Source: CAD feature listing. Evaluate the final solid. Frame: model axes, mm. Give positions to 0.01 mm unless a question says otherwise; leave off trailing zeros. Order: outer loops, then holes, each group sorted by start corner. A loop starts at its lowest first (then second) coordinate and runs counter-clockwise, first axis right, second up. Notation, with made-up numbers: M -37.75,31.25 L -9.75,31.25 A18 cw -9.75,48.25 Z; hole C 60.5,48.5 d3. An arc over 180 degrees is marked long. Return JSON: item names as keys, results as strings.
Autodesk Inventor part; units mm, degrees
ref_plane "YZ Plane" through (0, 0, 0) normal (1, 0, 0) x (0, 1, 0)
ref_plane "XZ Plane" through (0, 0, 0) normal (0, 1, 0) x (-1, 0, 0)
ref_plane "XY Plane" through (0, 0, 0) normal (0, 0, 1) x (1, 0, 0)
sketch "Sketch1" plane through (0, 0, 0) normal (0, 1, 0) x (-1, 0, 0)
  line L0 (-3.175, -3.175) -> (3.175, -3.175)
  line L1 (3.175, -3.175) -> (3.175, 3.175)
  line L2 (3.175, 3.175) -> (-3.175, 3.175)
  line L3 (-3.175, 3.175) -> (-3.175, -3.175)
  line L4 (-3.175, -3.175) -> (3.175, 3.175) construction
  line L5 (3.175, -3.175) -> (-3.175, 3.175) construction
  point P0 (0, 0)
  dimension "d0" = 6.35
  dimension "d1" = 6.35
extrude "Extrusion1" add sketch "Sketch1" along normal blind 68.58
fillet "Fillet1" radius 1.5875 4 edges at (3.175, 34.29, 3.175) (3.175, 34.29, -3.175) (-3.175, 34.29, -3.175) (-3.175, 34.29, 3.175)
fillet "Fillet2" radius 0.7937 16 edges at (2.71, 0, -2.71) (0, 0, -3.175) (-2.71, 0, -2.71) (-3.175, 0, 0) (-2.71, 0, 2.71) (0, 0, 3.175) (2.71, 0, 2.71) (3.175, 0, 0) (2.71, 68.58, -2.71) (0, 68.58, -3.175) (-2.71, 68.58, -2.71) (-3.175, 68.58, 0) (-2.71, 68.58, 2.71) (0, 68.58, 3.175) (2.71, 68.58, 2.71) (3.175, 68.58, 0)
sketch "Sketch2" plane through (-1.5875, 67.7863, 3.175) normal (0, 0, 1) x (1, 0, 0)
  circle A0 centre (1.5875, -64.6113) radius 1.9844
  line L0 (0, -67.7863) -> (3.175, -67.7863)
  point P0 (1.5875, -67.7863)
  dimension "d6" = 3.9688
  dimension "d7" = 3.175
extrude "Extrusion2" cut sketch "Sketch2" against normal blind 50.8
sketch "Sketch3" plane through (-1.5875, 67.7863, 3.175) normal (0, 0, 1) x (1, 0, 0)
  circle A0 centre (1.5875, -23.7173) radius 1.9844
  arc A1 (3.175, -63.4206) -> (0, -63.4206) centre (1.5875, -64.6113) ccw
  point P0 (1.5875, -67.7863)
  dimension "d10" = 3.9688
  dimension "d11" = 40.894
extrude "Extrusion3" cut sketch "Sketch3" against normal blind 50.8
properties part number "wedgec" material "Stainless Steel"
1. Section query C-C (z = -0.5). Return loops of the section in (x, y) (3 decimals).
Evaluation:
{"outline": "M -3.175,0.794 A0.794 ccw -2.381,0 L 2.381,0 A0.794 ccw 3.175,0.794 L 3.175,67.786 A0.794 ccw 2.381,68.58 L -2.381,68.58 A0.794 ccw -3.175,67.786 Z; hole C 0,3.175 d3.969; hole C 0,44.069 d3.969"}
2. First-contact query: pin 1 (3 mm diameter, centred on x = -0.5, z = 0.5, fed in from -Y). Flat tip, straight axial feed; report the tip coordinate or a pass-through.
Evaluation:
{"pin 1": "stops at y = 0"}
3. Section query A-A (x = 0.5). Return loops of the section in (y, z) (3 decimals).
Evaluation:
{"outline": "M 0,-2.381 A0.794 ccw 0.794,-3.175 L 1.255,-3.175 L 1.255,3.175 L 0.794,3.175 A0.794 ccw 0,2.381 Z; M 5.095,-3.175 L 42.149,-3.175 L 42.149,3.175 L 5.095,3.175 Z; M 45.989,-3.175 L 67.786,-3.175 A0.794 ccw 68.58,-2.381 L 68.58,2.381 A0.794 ccw 67.786,3.175 L 45.989,3.175 Z"}
4. Section query B-B (y = 11). Return loops of the section in (x, z) (1 decimal), then the cut area to 3 significant figures.
Evaluation:
{"outline": "M -3.2,-1.6 A1.6 ccw -1.6,-3.2 L 1.6,-3.2 A1.6 ccw 3.2,-1.6 L 3.2,1.6 A1.6 ccw 1.6,3.2 L -1.6,3.2 A1.6 ccw -3.2,1.6 Z", "area": "38.2 mm^2"}
5. Draft query along X for faces 1 (the face through (-0.43, 1.238, 0.044)), 2 (the face through (2.7, 34.76, 2.72)), 3 (the face through (0, 23, -3.175)). Return one class per face: pulls with the +X half, pulls with the -X half, needs draft (parallel to the pull), parting line crosses it, or undercut.
Evaluation:
{"face 1": "undercut", "face 2": "pulls with the +X half", "face 3": "needs draft"}
6. Ray query, probe 1 along Y at (x, z) = (1.75, -1.25); probe 2 along Y at (x, z) = (-1.25, 1.75); probe 3 along Z at (x, y) = (-1.75, 39.5). Return the intervals inside material, ascending.
Evaluation:
{"probe 1": "y = 0 to 2.24, 4.11 to 43.13, 45 to 68.58", "probe 2": "y = 0 to 1.63, 4.72 to 42.53, 45.61 to 68.58", "probe 3": "z = -3.17 to 3.17"}
